Verification items for the finished model (mm, model axes). A direction names the side the tool comes from. Round coordinates to 2 decimals unless told otherwise and drop trailing zeros. Loops run counter-clockwise (first coordinate to the right, second up) from the corner with the lowest first, then second, coordinate; pieces in that order, holes last. Notation, with made-up numbers: (-19.75, 20.25) -> (22.25, 20.25) arc R15 cw to (22.25, 42.25) -> close; hole circle Ø11 at (63, 74). An arc over 180 degrees is marked (long way). Use CSV: the item, a comma, the result in double quotes. Start each with the question number.
```python
from build123d import *

# Parameters (mm, degrees)
F1_DEPTH = 14.478
F2_R     = 1.27
F3_R     = 2.159
F4_DEPTH = 12.0914
F6_DEPTH = 14.479


with BuildPart() as f1:
    # F0 (on Front) → F1 (new body)
    with BuildSketch(Plane.XZ):
        Polygon((-18.2118, 4.4704), (0, 4.4704), (18.2118, 4.4704), (18.2118, 0), (30.9118, 0), (30.9118, 2.54), (35.9918, 2.54), (35.9918, 8.89), (30.9118, 8.89), (30.9118, 12.0904), (0, 12.0904), (-30.9118, 12.0904), (-30.9118, 8.89), (-35.9918, 8.89), (-35.9918, 2.54), (-30.9118, 2.54), (-30.9118, 0), (-18.2118, 0), align=None)
    extrude(amount=F1_DEPTH)

    # F2
    f2_edges = [f1.edges().sort_by_distance(p)[0] for p in [
        (-18.2118, -7.239, 4.4704),
        (18.2118, -7.239, 4.4704),
    ]]
    fillet(f2_edges, radius=F2_R)

    # F3 (on face) → F4 (cut, through all)
    with BuildSketch(Plane(origin=(0, 0, 0), x_dir=(1, 0, 0), z_dir=(0, 0, -1))):
        with Locations((-27.1018, 3.81)):
            Circle(F3_R)
        with Locations((27.1018, 3.81)):
            Circle(F3_R)
    extrude(amount=-F4_DEPTH, mode=Mode.SUBTRACT)

    # F5 (on face) → F6 (cut, through all)
    with BuildSketch(Plane(origin=(0, 0, 0), x_dir=(-1, 0, 0), z_dir=(0, 1, 0))):
        with BuildLine():
            Line((20.6248, 0), (24.6888, 0))
            ThreePointArc((24.6888, 0), (22.6568, 2.032), (20.6248, 0))
        make_face()
        with BuildLine():
            Line((-24.6888, 0), (-20.6248, 0))
            ThreePointArc((-20.6248, 0), (-22.6568, 2.032), (-24.6888, 0))
        make_face()
    extrude(amount=-F6_DEPTH, mode=Mode.SUBTRACT)


solid = f1.part
```
Q1. Cross-section at B-B (z = 1.25). Record the boundary of the cut face in (x, y), and give its area (3 significant figures).
Q2. Tool access check on faces 5 (the face through (33, -7, 8.89)), 6 (the face through (-17.83, -7.34, 4.11)), 7 (the face through (33, -7, 2.54)), 8 (the face through (-33, -7, 2.54)), 9 (the face through (-33, -7, 8.89)). Record the directions out of +Z, -Z, +X, -X, +Y, -Y that give a thin tool (end or side, any length) a straight path to the whole face; none if there is none.
Q3. Cross-section at D-D (z = 11.25). Record the boundary of the cut face in (x, y).
Q4. Depth check by flat-ended pin: pin 1 Ø4 at (x, y) = (-32.5, -10.5) entering from -Z; pin 2 Ø4 at (x, y) = (33, -6.5) entering from +Z; pin 3 Ø7 at (x, y) = (5.5, -10.5) entering from -Z; pin 4 Ø1.6 at (y, z) = (-8, 1) entering from +X. Enter the tip coordinate at first touch or a pass-through.
Q5. Cross-section at C-C (y = -9). Record the boundary of the cut face in (x, z), and give its area (3 significant figures).
Q6. Thickness scan on L1, parallel to X at y = -3.81, z = 5; L2, parallel to X at y = -4, z = 7; L3, parallel to X at y = -3.81, z = 4. Record the ranges inside material, lowest first. Write a range as from..to.
Q7. Release check for a two-part mould opening along X. For faces 1 (the face through (18.212, -7, 2)), 2 (the face through (30.912, -7, 1)), 3 (the face through (-30.912, -7, 11)), 4 (the face through (29.096, -2.983, 5.961)) record: +X half, -X half, draft (parallel to the pull), parting line (faces both ways), or undercut.
Q8. Cross-section at A-A (y = -3.81). State how many separate pieces and enclosed holes the cut face has, and give its area (3 significant figures).
Answer list:
1,outline,"(-30.91, -14.48) -> (-24.26, -14.48) -> (-24.26, 0) -> (-30.91, 0) -> close; (-21.05, -14.48) -> (-18.21, -14.48) -> (-18.21, 0) -> (-21.05, 0) -> close; (18.21, -14.48) -> (21.05, -14.48) -> (21.05, 0) -> (18.21, 0) -> close; (24.26, -14.48) -> (30.91, -14.48) -> (30.91, 0) -> (24.26, 0) -> close; hole circle Ø4.32 at (-27.1, -3.81); hole circle Ø4.32 at (27.1, -3.81)"
1,area,"246 mm2"
2,face 5,"+Z, +X, +Y, -Y"
2,face 6,"-Z, +Y, -Y"
2,face 7,"-Z, +X, +Y, -Y"
2,face 8,"-Z, -X, +Y, -Y"
2,face 9,"+Z, -X, +Y, -Y"
3,outline,"(-30.91, -14.48) -> (30.91, -14.48) -> (30.91, 0) -> (-30.91, 0) -> close; hole circle Ø4.32 at (-27.1, -3.81); hole circle Ø4.32 at (27.1, -3.81)"
4,pin 1,"stops at z = 0"
4,pin 2,"stops at z = 8.89"
4,pin 3,"stops at z = 4.47"
4,pin 4,"stops at x = 30.91"
5,outline,"(-35.99, 2.54) -> (-30.91, 2.54) -> (-30.91, 0) -> (-24.69, 0) arc R2.03 cw to (-20.62, 0) -> (-18.21, 0) -> (-18.21, 3.2) arc R1.27 cw to (-16.94, 4.47) -> (16.94, 4.47) arc R1.27 cw to (18.21, 3.2) -> (18.21, 0) -> (20.62, 0) arc R2.03 cw to (24.69, 0) -> (30.91, 0) -> (30.91, 2.54) -> (35.99, 2.54) -> (35.99, 8.89) -> (30.91, 8.89) -> (30.91, 12.09) -> (-30.91, 12.09) -> (-30.91, 8.89) -> (-35.99, 8.89) -> close"
5,area,"637 mm2"
6,L1,"x = -35.99..-29.26, -24.94..24.94, 29.26..35.99"
6,L2,"x = -35.99..-29.25, -24.95..24.95, 29.25..35.99"
6,L3,"x = -35.99..-29.26, -24.94..-17.93, 17.93..24.94, 29.26..35.99"
7,face 1,"undercut"
7,face 2,"+X half"
7,face 3,"-X half"
7,face 4,"undercut"
8,separate pieces,"3"
8,enclosed holes,"0"
8,area,"532 mm2"
